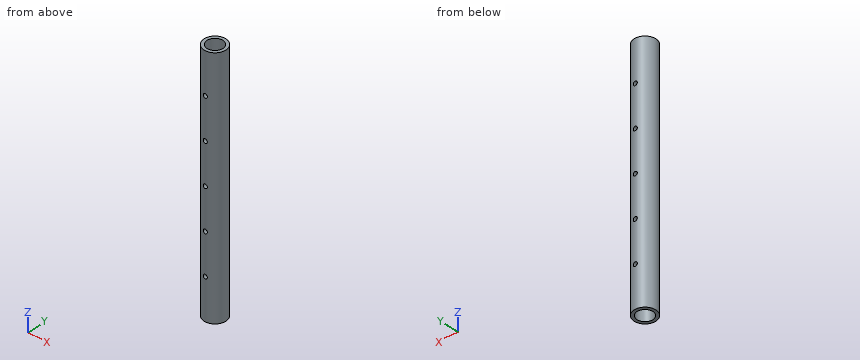
from build123d import *

# Parameters (mm, degrees)
F0_R          = 10.16
F0_R_2        = 7.366
F1_DEPTH      = 228.6
F2_R          = 1.905
F3_DEPTH      = 25.4
F3_DEPTH_BACK = 25.4


with BuildPart() as f1:
    # F0 (on Top) → F1 (new body)
    with BuildSketch(Plane.XY):
        Circle(F0_R)
        Circle(F0_R_2, mode=Mode.SUBTRACT)
    extrude(amount=F1_DEPTH)

    # F2 (on Front) → F3 (cut, two sides)
    with BuildSketch(Plane.XZ) as f3_sk:
        with Locations((0, 38.1)):
            Circle(F2_R)
        with Locations((0, 76.2)):
            Circle(F2_R)
        with Locations((0, 114.3)):
            Circle(F2_R)
        with Locations((0, 152.4)):
            Circle(F2_R)
        with Locations((0, 190.5)):
            Circle(F2_R)
    extrude(amount=-F3_DEPTH, mode=Mode.SUBTRACT)
    extrude(f3_sk.sketch, amount=F3_DEPTH_BACK, mode=Mode.SUBTRACT)


solid = f1.part
Work out the finished part from the listing and answer in its coordinate system (mm). Coordinates: 2 decimals unless noted, no trailing zeros. Write each loop counter-clockwise with the first axis right and the second up, starting at its lowest first coordinate (ties: lowest second). Pieces come first, ordered by that corner, then holes. Notation, with made-up numbers: M 81.25,11 L 91.25,11 A21 cw 91.25,50 Z; hole C 12,15 d11. An arc over 180 degrees is marked long. Write item = value, one per line.
1. Flat-ended cylindrical pins translate along their axes: pin 1 (5 mm diameter, centred on x = 0, z = 38.1, fed in from -Y); pin 2 (3 mm diameter, centred on x = 0, z = 190.5, fed in from -Y); pin 3 (1 mm diameter, centred on y = -1.5, z = 86.5, fed in from -X); pin 4 (1.5 mm diameter, centred on y = -3.5, z = 151, fed in from +X). Find the tip coordinate at first contact, or state that the pin passes through.
Solution:
pin_1 = -10.16
pin_2 = through
pin_3 = -10.11
pin_4 = 9.78
2. The part is cut by section C-C (x = 0). State how many separate pieces and enclosed holes the cut face has, then the cut area to 3 significant figures.
Solution:
separate_pieces = 12
enclosed_holes = 0
area = 1,170 mm2
3. The part is cut by section A-A (y = 4.75). Determine the outline of the cut face in (x, z).
Solution:
outline = M -8.98,0 L -5.63,0 L -5.63,228.6 L -8.98,228.6 Z; M 5.63,0 L 8.98,0 L 8.98,228.6 L 5.63,228.6 Z
4. The part is cut by section B-B (z = 190.5). Determine the outline of the cut face in (x, y) (3 decimals), then the cut area to 3 significant figures.
Solution:
outline = M -1.905,-9.98 L -1.905,-7.115 A7.366 cw -1.905,7.115 L -1.905,9.98 A10.16 ccw Z; M 1.905,-9.98 A10.16 ccw 1.905,9.98 L 1.905,7.115 A7.366 cw 1.905,-7.115 Z
area = 132 mm2
5. The part is cut by section D-D (z = 130). Determine the outline of the cut face in (x, y), then the cut area to 3 significant figures.
Solution:
outline = C 0,0 d20.32; hole C 0,0 d14.73
area = 154 mm2
6. Straight lines are drawn through the part: line 1 (Z direction, x = 0, y = -7.85) (3 decimals); line 2 (Y direction, x = 0.75, z = 197); line 3 (Y direction, x = 0, z = 69.5). For each, find the intervals that lie inside material, in ascending order. Write a range as from..to.
Solution:
line_1 = 0..36.195, 40.005..74.295, 78.105..112.395, 116.205..150.495, 154.305..188.595, 192.405..228.6
line_2 = -10.13..-7.33, 7.33..10.13
line_3 = -10.16..-7.37, 7.37..10.16
